Could you check a few things on this model? Use its own coordinates, in mm. Face numbers are marked on the shaded views. Give positions to 0.01 mm unless a question says otherwise; leave off trailing zeros. Write each loop counter-clockwise with the first axis right and the second up, starting at its lowest first coordinate (ties: lowest second). Pieces come first, ordered by that corner, then holes. Notation, with made-up numbers: M 7,-5 L 44,-5 A18 ccw 44,6 Z; hole C -16.75,72.5 d4. An arc over 180 degrees is marked long. Use one line per item in the form item = value.
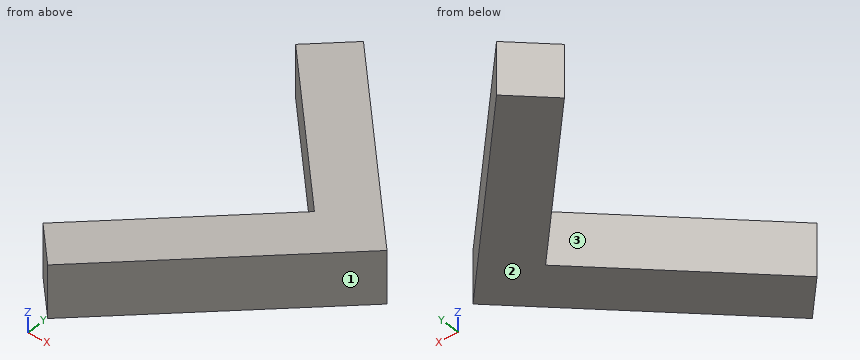
from build123d import *

# Parameters (mm, degrees)
BOX081_W               = 1
BOX081_H               = 5
BOX081_DEPTH           = 1
BOX081_PLACEMENT_ANGLE = 45
BOX084_W               = 1
BOX084_H               = 4
BOX084_DEPTH           = 1
BOX084_PLACEMENT_ANGLE = 135


with BuildPart() as cube081:
    # Box081 → Box081 (new body)
    with BuildSketch(Plane.XY):
        with Locations((0.5, 2.5)):
            Rectangle(BOX081_W, BOX081_H)
    extrude(amount=BOX081_DEPTH)


with BuildPart() as cube081_1:
    # Box081 placement: moved
    add(cube081.part.rotate(Axis((0, 0, 0), (0, 0, 1)), BOX081_PLACEMENT_ANGLE))


with BuildPart() as obj1:
    # Box084 → Box084 (new body)
    with BuildSketch(Plane.XY):
        with Locations((0.5, 2)):
            Rectangle(BOX084_W, BOX084_H)
    extrude(amount=BOX084_DEPTH)


with BuildPart() as obj1_1:
    # Box084 placement: moved
    add(obj1.part.rotate(Axis((0, 0, 0), (0, 0, 1)), BOX084_PLACEMENT_ANGLE))

    # Fusion015: union Cube081
    add(cube081_1.part)


with BuildPart() as obj1_2:
    # Fusion015 placement: moved
    add(obj1_1.part.moved(Location((16, 5, 0))))


solid = obj1_2.part
1) I want a section at C-C, the plane x = 15.95. Please give me the cut outline in (y, z), plus the area to 3 significant figures.
Checked values:
outline = M 4.95,0 L 6.46,0 L 6.46,1 L 4.95,1 Z
area = 1.51 mm2
2) I want a section at D-D, the plane y = 4.75. Please give me the cut outline in (x, z).
Checked values:
outline = M 14.34,0 L 15.75,0 L 15.75,1 L 14.34,1 Z
3) Thinking about a two-plate mould opening in Y: for the marked faces 1, 2 and 3, which applies, released by +Y, released by -Y, zero draft, split by the parting line, or undercut?
Checked values:
face_1 = released by -Y
face_2 = zero draft
face_3 = undercut
4) I want a section at A-A, the plane x = 14.25. Please give me the cut outline in (y, z), plus the area to 3 significant figures.
Checked values:
outline = M 3.25,0 L 4.66,0 L 4.66,1 L 3.25,1 Z; M 6.75,0 L 8.16,0 L 8.16,1 L 6.75,1 Z
area = 2.83 mm2
5) If I drill on L1, parallel to Y at x = 13.7, z = 0.65; L2, parallel to Y at x = 15.15, z = 0.95; L3, parallel to X at y = 7.5, z = 0.35, over which ranges is the centre line in solid material (lowest first)?
Checked values:
L1 = 2.7 to 4.11, 7.3 to 8.71
L2 = 4.15 to 5.56, 5.85 to 7.26
L3 = 13.5 to 14.91
6) I want a section at B-B, the plane z = 0.35. Please give me the cut outline in (x, y).
Checked values:
outline = M 12.46,2.88 L 13.17,2.17 L 16.71,5.71 L 13.17,9.24 L 12.46,8.54 L 15.29,5.71 Z
